Input: part model. Units: mm. Frame: model coordinates. Face numbers are marked on the shaded views. A direction names the side the tool comes from. Give positions to 0.01 mm unless a question says otherwise; leave off trailing zeros. Loops run counter-clockwise (first coordinate to the right, second up) from the corner with the lowest first, then second, coordinate; pieces in that order, holes last. Notation, with made-up numbers: (15.25, -11.5) -> (29.25, -11.5) arc R16 ccw to (29.25, 5.5) -> close; hole circle Ø11 at (24.25, 40). An arc over 180 degrees is marked (long way). One line per question, with ' | ' between items.
from build123d import *

# Parameters (mm, degrees)
SKETCH1_W           = 0.5
SKETCH1_H           = 0.5
BOSS_EXTRUDE1_DEPTH = 10
SKETCH2_W           = 27
SKETCH2_H           = 10
SKETCH2_R           = 1.75
BOSS_EXTRUDE2_DEPTH = 5
SKETCH3_W           = 10
SKETCH3_H           = 8
CUT_EXTRUDE3_DEPTH  = 2
FILLET1_R           = 0.1
FILLET2_R           = 0.1


with BuildPart() as part:
    # Sketch1 → Boss-Extrude1 (new body)
    with BuildSketch(Plane.XY):
        Polygon((20, 0), (0, 0), (0, -10), (20, -10), (20, -7.45), (19.5, -7.45), (4.4, -7.45), (4.4, -2.55), (19.5, -2.55), (20, -2.55), align=None)
        with Locations((19.75, -7.2)):
            Rectangle(SKETCH1_W, SKETCH1_H)
        with Locations((19.75, -2.8)):
            Rectangle(SKETCH1_W, SKETCH1_H)
    extrude(amount=BOSS_EXTRUDE1_DEPTH)

    # Sketch2 → Boss-Extrude2 (add)
    with BuildSketch(Plane.XY.offset(10)):
        with Locations((-13.5, -5)):
            Rectangle(SKETCH2_W, SKETCH2_H)
        with Locations((-23, -5)):
            Circle(SKETCH2_R, mode=Mode.SUBTRACT)
        with Locations((-4, -5)):
            Circle(SKETCH2_R, mode=Mode.SUBTRACT)
    extrude(amount=-BOSS_EXTRUDE2_DEPTH)

    # Sketch3 → Cut-Extrude3 (cut)
    with BuildSketch(Plane.XY.offset(10)):
        with Locations((-13.5, -5)):
            Rectangle(SKETCH3_W, SKETCH3_H)
    extrude(amount=-CUT_EXTRUDE3_DEPTH, mode=Mode.SUBTRACT)

    # Fillet1
    fillet1_edges = [part.edges().sort_by_distance(p)[0] for p in [
        (19.5, -7.45, 5),
        (19.5, -2.55, 5),
    ]]
    fillet(fillet1_edges, radius=FILLET1_R)

    # Fillet2
    fillet2_edges = [part.edges().sort_by_distance(p)[0] for p in [
        (19.5, -6.95, 5),
        (20, -6.95, 5),
        (20, -3.05, 5),
        (19.5, -3.05, 5),
    ]]
    fillet(fillet2_edges, radius=FILLET2_R)


solid = part.part
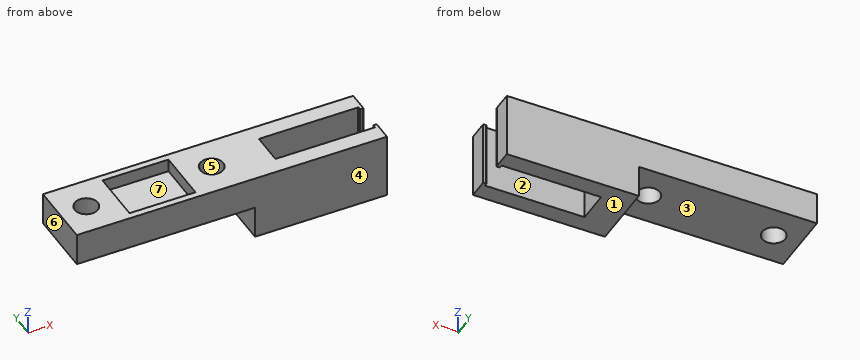
1. Section query A-A (x = 12). Output: boundary loops of the cut face in (y, z).
Determined:
outline: (-10, 0) -> (-7.45, 0) -> (-7.45, 10) -> (-10, 10) -> close; (-2.55, 0) -> (0, 0) -> (0, 10) -> (-2.55, 10) -> close
2. Pin query (flat end, axial travel): P1, Ø5, axis at x = -17, y = -3, coming from the -Z side; P2, Ø4, axis at x = -14, y = -6.5, coming from the +Z side; P3, Ø1.5, axis at y = -6, z = 3.5, coming from the -X side. Return the tip coordinate at first contact, or that it passes through.
Determined:
P1: stops at z = 5 | P2: stops at z = 8 | P3: stops at x = 0
3. Section query D-D (z = 1.75). Output: boundary loops of the cut face in (x, y).
Determined:
outline: (0, -10) -> (20, -10) -> (20, -7.05) arc R0.1 ccw to (19.9, -6.95) -> (19.6, -6.95) arc R0.1 ccw to (19.5, -7.05) -> (19.5, -7.35) arc R0.1 cw to (19.4, -7.45) -> (4.4, -7.45) -> (4.4, -2.55) -> (19.4, -2.55) arc R0.1 cw to (19.5, -2.65) -> (19.5, -2.95) arc R0.1 ccw to (19.6, -3.05) -> (19.9, -3.05) arc R0.1 ccw to (20, -2.95) -> (20, 0) -> (0, 0) -> close
4. Section query C-C (x = -11.5). Output: boundary loops of the cut face in (y, z).
Determined:
outline: (-10, 5) -> (0, 5) -> (0, 10) -> (-1, 10) -> (-1, 8) -> (-9, 8) -> (-9, 10) -> (-10, 10) -> close
5. Section query B-B (y = -5). Output: boundary loops of the cut face in (x, z).
Determined:
outline: (-27, 5) -> (-24.75, 5) -> (-24.75, 10) -> (-27, 10) -> close; (-21.25, 5) -> (-5.75, 5) -> (-5.75, 10) -> (-8.5, 10) -> (-8.5, 8) -> (-18.5, 8) -> (-18.5, 10) -> (-21.25, 10) -> close; (-2.25, 5) -> (0, 5) -> (0, 0) -> (4.4, 0) -> (4.4, 10) -> (-2.25, 10) -> close
6. Pull-direction query (X, two-part tool) for the marked faces 4, 5, 6 and 7; classes: pulls with the +X half, pulls with the -X half, needs draft (parallel to the pull), parting line crosses it, or undercut.
Determined:
face 4: needs draft | face 5: undercut | face 6: pulls with the -X half | face 7: undercut
7. Ray query, line 1 along Y through (x, z) = (-23, 7.5); line 2 along X through (y, z) = (-7.5, 9); line 3 along X through (y, z) = (-6, 9.25). Return the intervals inside material, ascending. Write a range as from..to.
Determined:
line 1: y = -10..-6.75, -3.25..0 | line 2: x = -27..-18.5, -8.5..20 | line 3: x = -27..-24.44, -21.56..-18.5, -8.5..-5.44, -2.56..4.4
8. Reachability of the marked faces 1, 2 and 3 from +Z, -Z, +X, -X, +Y, -Y: full face, straight path, thin tool, end or side. Return the list, or none.
Determined:
face 1: -Z, +X, -X, +Y, -Y | face 2: +Z, -Z | face 3: -Z, -X, +Y, -Y
